from build123d import *

# Parameters (mm, degrees)
F_01_COMMON_SLIDER_BLANK_DEPTH                 = 9
F_02_START                                     = -0.5
S02_ROUND_LOCATING_GUIDE_AND_RELIEVED_R        = 2.75
F_02_ROUND_LOCATING_GUIDE_AND_RELIEVED_C_DEPTH = 10
F_03_START                                     = -0.5
S03_THREE_DROP_IN_SPRING_SEATS_W               = 16.6
S03_THREE_DROP_IN_SPRING_SEATS_H               = 9.3
F_03_THREE_DROP_IN_SPRING_SEATS_DEPTH          = 10
F_04_START                                     = -0.5
S04_KEEPER_SCREW_HOLES_R                       = 1.7
F_04_KEEPER_SCREW_HOLES_DEPTH                  = 10
F_07_START                                     = -0.15
S07_CLEARANCE_TUNNEL_FOR_ROTATING_SPIN_R       = 5.2
F_07_CLEARANCE_TUNNEL_FOR_ROTATING_SPIND_DEPTH = 109.311915664
SKETCH1_R                                      = 1.75
SKETCH1_R_2                                    = 1.75028584
CUT_EXTRUDE1_DEPTH                             = 10


with BuildPart() as part:
    # S01 - Common slider blank → 01 - Common slider blank (new body)
    with BuildSketch(Plane.XY):
        with BuildLine():
            Line((-43, -97), (43, -97))
            ThreePointArc((43, -97), (45.828427125, -95.828427125), (47, -93))
            Line((47, -93), (47, -55))
            ThreePointArc((47, -55), (45.828427125, -52.171572875), (43, -51))
            Line((43, -51), (-43, -51))
            ThreePointArc((-43, -51), (-45.828427125, -52.171572875), (-47, -55))
            Line((-47, -55), (-47, -93))
            ThreePointArc((-47, -93), (-45.828427125, -95.828427125), (-43, -97))
        make_face()
    extrude(amount=F_01_COMMON_SLIDER_BLANK_DEPTH)

    # S02 - Round locating guide and relieved companion → 02 - Round locating guide and relieved companion (cut)
    with BuildSketch(Plane.XY.offset(F_02_START)):
        with Locations((-32, -83)):
            Circle(S02_ROUND_LOCATING_GUIDE_AND_RELIEVED_R)
        with BuildLine():
            Line((31.6, -80.25), (32.4, -80.25))
            ThreePointArc((32.4, -80.25), (35.15, -83), (32.4, -85.75))
            Line((32.4, -85.75), (31.6, -85.75))
            ThreePointArc((31.6, -85.75), (28.85, -83), (31.6, -80.25))
        make_face()
    extrude(amount=F_02_ROUND_LOCATING_GUIDE_AND_RELIEVED_C_DEPTH, mode=Mode.SUBTRACT)

    # S03 - Three drop-in spring seats → 03 - Three drop-in spring seats (cut)
    with BuildSketch(Plane.XY.offset(F_03_START)):
        with Locations((-25.980762114, -54.65)):
            Rectangle(S03_THREE_DROP_IN_SPRING_SEATS_W, S03_THREE_DROP_IN_SPRING_SEATS_H)
        with Locations((25.980762114, -54.65)):
            Rectangle(S03_THREE_DROP_IN_SPRING_SEATS_W, S03_THREE_DROP_IN_SPRING_SEATS_H)
        with Locations((0, -54.65)):
            Rectangle(S03_THREE_DROP_IN_SPRING_SEATS_W, S03_THREE_DROP_IN_SPRING_SEATS_H)
    extrude(amount=F_03_THREE_DROP_IN_SPRING_SEATS_DEPTH, mode=Mode.SUBTRACT)

    # S04 - Keeper screw holes → 04 - Keeper screw holes (cut)
    with BuildSketch(Plane.XY.offset(F_04_START)):
        with Locations((-41, -58.3)):
            Circle(S04_KEEPER_SCREW_HOLES_R)
        with Locations((41, -58.3)):
            Circle(S04_KEEPER_SCREW_HOLES_R)
    extrude(amount=F_04_KEEPER_SCREW_HOLES_DEPTH, mode=Mode.SUBTRACT)

    # S07 - Clearance tunnel for rotating spindle retainer → 07 - Clearance tunnel for rotating spindle retainer (cut, through all)
    with BuildSketch(Plane.XY.offset(F_07_START)):
        with Locations((0, -82)):
            Circle(S07_CLEARANCE_TUNNEL_FOR_ROTATING_SPIN_R)
    extrude(amount=F_07_CLEARANCE_TUNNEL_FOR_ROTATING_SPIND_DEPTH, mode=Mode.SUBTRACT)

    # Sketch1 → Cut-Extrude1 (cut)
    with BuildSketch(Plane.XY.offset(9)):
        with Locations((8, -82)):
            Circle(SKETCH1_R)
        with Locations((0, -74)):
            Circle(SKETCH1_R)
        with Locations((0, -90)):
            Circle(SKETCH1_R)
        with Locations((-8, -82)):
            Circle(SKETCH1_R_2)
    extrude(amount=-CUT_EXTRUDE1_DEPTH, mode=Mode.SUBTRACT)


solid = part.part
The listing builds one solid part. Answer for the finished solid, in the listing's coordinates (mm). A direction names the side the tool comes from. Round coordinates to 2 decimals unless told otherwise and drop trailing zeros. Loops run counter-clockwise (first coordinate to the right, second up) from the corner with the lowest first, then second, coordinate; pieces in that order, holes last. Notation, with made-up numbers: M 12.25,-8 L 18.25,-8 A15 cw 18.25,11 Z; hole C 32.5,0 d11. An arc over 180 degrees is marked long. Return JSON: item names as keys, results as strings.
Q1. The mould has two halves that part along Y. Classify faces 1 (the face through (-45.797, -52.141, 4.437)), 2 (the face through (28.85, -83.06, 4.44)), 3 (the face through (-8.3, -55, 4)): released by +Y, released by -Y, zero draft, split by the parting line, or undercut.
Results list:
{"face 1": "released by +Y", "face 2": "undercut", "face 3": "zero draft"}
Q2. Find section A-A, the plane y = -58.3. Determine the outline of the cut face in (x, z), plus the area to 3 significant figures.
Results list:
{"outline": "M -47,0 L -42.7,0 L -42.7,9 L -47,9 Z; M -39.3,0 L -34.28,0 L -34.28,9 L -39.3,9 Z; M -17.68,0 L -8.3,0 L -8.3,9 L -17.68,9 Z; M 8.3,0 L 17.68,0 L 17.68,9 L 8.3,9 Z; M 34.28,0 L 39.3,0 L 39.3,9 L 34.28,9 Z; M 42.7,0 L 47,0 L 47,9 L 42.7,9 Z", "area": "337 mm2"}
Q3. Each of these flat-tipped pins is pushed along its axis until it touches: pin 1 Ø2.5 at (x, z) = (-28, 4.5) entering from +Y; pin 2 Ø4.5 at (x, y) = (-32, -83) entering from -Z; pin 3 Ø5.5 at (x, y) = (41, -58.3) entering from +Z. Where does it stop, or does it pass through?
Results list:
{"pin 1": "stops at y = -59.3", "pin 2": "passes through", "pin 3": "stops at z = 9"}
Q4. Find section B-B, the plane x = -32. Determine the outline of the cut face in (y, z).
Results list:
{"outline": "M -97,0 L -85.75,0 L -85.75,9 L -97,9 Z; M -80.25,0 L -59.3,0 L -59.3,9 L -80.25,9 Z"}
Q5. Find section C-C, the plane y = -90. Determine the outline of the cut face in (x, z), plus the area to 4 significant figures.
Results list:
{"outline": "M -47,0 L -1.75,0 L -1.75,9 L -47,9 Z; M 1.75,0 L 47,0 L 47,9 L 1.75,9 Z", "area": "814.5 mm2"}
Q6. Find the intervals of material crossed by line 1 along X through (y, z) = (-56.5, 0.5); line 2 along Y through (x, z) = (0, 4); line 3 along X through (y, z) = (-82, 3.25), in increasing order. Write a range as from..to.
Results list:
{"line 1": "x = -47..-34.28, -17.68..-8.3, 8.3..17.68, 34.28..47", "line 2": "y = -97..-91.75, -88.25..-87.2, -76.8..-75.75, -72.25..-59.3", "line 3": "x = -47..-34.56, -29.44..-9.75, -6.25..-5.2, 5.2..6.25, 9.75..29.04, 34.96..47"}
Q7. Find section D-D, the plane y = -82. Determine the outline of the cut face in (x, z).
Results list:
{"outline": "M -47,0 L -34.56,0 L -34.56,9 L -47,9 Z; M -29.44,0 L -9.75,0 L -9.75,9 L -29.44,9 Z; M -6.25,0 L -5.2,0 L -5.2,9 L -6.25,9 Z; M 5.2,0 L 6.25,0 L 6.25,9 L 5.2,9 Z; M 9.75,0 L 29.04,0 L 29.04,9 L 9.75,9 Z; M 34.96,0 L 47,0 L 47,9 L 34.96,9 Z"}
Q8. Which of the six approach directions +Z, -Z, +X, -X, +Y, -Y give full straight-line access (tool end or side, diameter ignored) to faces 4 (the face through (39, -51, 4)), 5 (the face through (34.281, -55, 4))?
Results list:
{"face 4": "+Z, -Z, +X, -X, +Y", "face 5": "+Z, -Z, +Y"}
